Could you check a few things on this model? Use its own coordinates, in mm. A direction names the side the tool comes from. Give positions to 0.01 mm unless a question says otherwise; leave off trailing zeros. Loops run counter-clockwise (first coordinate to the right, second up) from the corner with the lowest first, then second, coordinate; pieces in that order, holes last. Notation, with made-up numbers: (19.25, 52) - (55.25, 52) arc R31 cw to (55.25, 86) - close; hole circle Ø5 at (47, 1.25). An arc over 180 degrees is marked (long way). Use CSV: the item, a comma, the result in double quotes.
from build123d import *

# Parameters (mm, degrees)
SZKIC1_W                                = 77
SZKIC1_H                                = 40
SZKIC1_R                                = 1.5
DODANIE_WYCI_GNI_CIE1_DEPTH             = 2
SZKIC2_W                                = 77
SZKIC2_H                                = 40
SZKIC2_W_2                              = 73
SZKIC2_H_2                              = 36
DODANIE_WYCI_GNI_CIE2_DEPTH             = 19
WYTNIJ_WYCI_GNI_CIE1_DEPTH              = 60.356970947
ZAOKR_GLENIE1_R                         = 2.5
SZKIC4_W                                = 77
SZKIC4_H                                = 1
DODANIE_WYCI_GNI_CIE3_DEPTH             = 10
SZKIC5_W                                = 6
SZKIC5_H                                = 10
DODANIE_WYCI_GNI_CIE4_DEPTH             = 5
ZAOKR_GLENIE2_R                         = 2.5
ZAOKR_GLENIE2_OF_LUSTRO1_R              = 2.5
LUSTRO2_START                           = -13
LUSTRO2_DEPTH                           = 6
LUSTRO2_START_2                         = 7
LUSTRO2_2_DEPTH                         = 6
DODANIE_WYCI_GNI_CIE5_REACH             = 50.2
SZKIC6_R                                = 8.7
DODANIE_WYCI_GNI_CIE5_DIRECTION_2_REACH = 50.2
ZAOKR_GLENIE3_R                         = 0.5


# Read off the part's stored shape, not the designer's step: Lustro2
with BuildPart() as part:
    # Szkic1 → Dodanie-wyciągnięcie1 (new body)
    with BuildSketch(Plane(origin=(0, 0, 0), x_dir=(1, 0, 0), z_dir=(0, 1, 0))):
        Rectangle(SZKIC1_W, SZKIC1_H)
        with Locations(Location((27.5, 9.5, 0), (0, 0, 270))):
            Circle(SZKIC1_R, mode=Mode.SUBTRACT)
        with Locations(Location((27.5, -9.5, 0), (0, 0, 90))):
            Circle(SZKIC1_R, mode=Mode.SUBTRACT)
        with Locations(Location((-27.5, -9.5, 0), (0, 0, 270))):
            Circle(SZKIC1_R, mode=Mode.SUBTRACT)
        with Locations(Location((-27.5, 9.5, 0), (0, 0, 90))):
            Circle(SZKIC1_R, mode=Mode.SUBTRACT)
    extrude(amount=DODANIE_WYCI_GNI_CIE1_DEPTH)

    # Szkic2 → Dodanie-wyciągnięcie2 (add)
    with BuildSketch(Plane(origin=(0, 2, 0), x_dir=(1, 0, 0), z_dir=(0, 1, 0))):
        Rectangle(SZKIC2_W, SZKIC2_H)
        Rectangle(SZKIC2_W_2, SZKIC2_H_2, mode=Mode.SUBTRACT)
    extrude(amount=DODANIE_WYCI_GNI_CIE2_DEPTH)

    # Szkic3 → Wytnij-wyciągnięcie1 (cut, through all)
    with BuildSketch(Plane.XY.offset(20)):
        Polygon((-12.5, 7.396479256), (12.5, 7.396479256), (12.5, 12.396479256), (25.5, 12.396479256), (25.5, 17.396479256), (36.5, 17.396479256), (36.5, 21), (-36.5, 21), (-36.5, 17.396479256), (-25.5, 17.396479256), (-25.5, 12.396479256), (-12.5, 12.396479256), align=None)
    extrude(amount=-WYTNIJ_WYCI_GNI_CIE1_DEPTH, mode=Mode.SUBTRACT)

    # Zaokrąglenie1
    zaokr_glenie1_edges = [part.edges().sort_by_distance(p)[0] for p in [
        (36.5, 17.396479256, 19),
        (25.5, 17.396479256, 19),
        (25.5, 12.396479256, 19),
        (12.5, 12.396479256, 19),
        (12.5, 7.396479256, 19),
        (-36.5, 17.396479256, 19),
        (-25.5, 17.396479256, 19),
        (-25.5, 12.396479256, 19),
        (-12.5, 12.396479256, 19),
        (-12.5, 7.396479256, 19),
        (12.5, 7.396479256, -19),
        (12.5, 12.396479256, -19),
        (25.5, 12.396479256, -19),
        (36.5, 17.396479256, -19),
        (25.5, 17.396479256, -19),
        (-12.5, 7.396479256, -19),
        (-12.5, 12.396479256, -19),
        (-36.5, 17.396479256, -19),
        (-25.5, 17.396479256, -19),
        (-25.5, 12.396479256, -19),
    ]]
    fillet(zaokr_glenie1_edges, radius=ZAOKR_GLENIE1_R - 0.0001)  # a hair under: the kernel refuses the full size

    # Szkic4 → Dodanie-wyciągnięcie3 (add)
    with BuildSketch(Plane(origin=(0, 2, 0), x_dir=(1, 0, 0), z_dir=(0, 1, 0))):
        Rectangle(SZKIC4_W, SZKIC4_H)
    extrude(amount=DODANIE_WYCI_GNI_CIE3_DEPTH)

    # Szkic5 → Dodanie-wyciągnięcie4 (add)
    with BuildSketch(Plane(origin=(-36.5, 0, 0), x_dir=(0, 0, -1), z_dir=(1, 0, 0))):
        with Locations((-10, 9.5)):
            Rectangle(SZKIC5_W, SZKIC5_H)
    dodanie_wyci_gni_cie4 = extrude(amount=DODANIE_WYCI_GNI_CIE4_DEPTH)

    # Zaokrąglenie2
    zaokr_glenie2_edges = [part.edges().sort_by_distance(p)[0] for p in [
        (-31.5, 14.5, 10),
    ]]
    fillet(zaokr_glenie2_edges, radius=ZAOKR_GLENIE2_R)

    # Lustro1: Dodanie-wyciągnięcie4 across plane
    add(dodanie_wyci_gni_cie4.mirror(Plane.XY))

    # Zaokrąglenie2 of Lustro1
    zaokr_glenie2_of_lustro1_edges = [part.edges().sort_by_distance(p)[0] for p in [
        (-31.5, 14.5, -10),
    ]]
    fillet(zaokr_glenie2_of_lustro1_edges, radius=ZAOKR_GLENIE2_OF_LUSTRO1_R)

    # Lustro2 outline → Lustro2 (add)
    with BuildSketch(Plane.XY.offset(LUSTRO2_START)):
        with BuildLine():
            Line((36.5, 14.5), (34, 14.5))
            ThreePointArc((34, 14.5), (32.232233047, 13.767766953), (31.5, 12))
            Line((31.5, 12), (31.5, 4.5))
            Line((31.5, 4.5), (36.5, 4.5))
            Line((36.5, 4.5), (36.5, 14.5))
        make_face()
    extrude(amount=LUSTRO2_DEPTH)

    # Lustro2 2 outline → Lustro2 2 (add)
    with BuildSketch(Plane.XY.offset(LUSTRO2_START_2)):
        with BuildLine():
            Line((36.5, 14.5), (34, 14.5))
            ThreePointArc((34, 14.5), (32.232233047, 13.767766953), (31.5, 12))
            Line((31.5, 12), (31.5, 4.5))
            Line((31.5, 4.5), (36.5, 4.5))
            Line((36.5, 4.5), (36.5, 14.5))
        make_face()
    extrude(amount=LUSTRO2_2_DEPTH)

    # Dodanie-wyciągnięcie5: up to this face of the body (flat: up to its plane)
    dodanie_wyci_gni_cie5_end = Plane(part.part.faces().sort_by_distance((31.5, 8.25, 10))[0])
    # Szkic6 → Dodanie-wyciągnięcie5 (add, up to the picked face)
    with BuildSketch(Plane(origin=(0, 0, 0), x_dir=(0, 0, -1), z_dir=(1, 0, 0)), mode=Mode.PRIVATE) as dodanie_wyci_gni_cie5_sk1:
        with Locations(Location((-9.25, 11, 0), (0, 0, 180))):
            Circle(SZKIC6_R)
    dodanie_wyci_gni_cie5_tool1 = split(extrude(dodanie_wyci_gni_cie5_sk1.sketch, amount=DODANIE_WYCI_GNI_CIE5_REACH, mode=Mode.PRIVATE), bisect_by=dodanie_wyci_gni_cie5_end, keep=Keep.BOTH, mode=Mode.PRIVATE)
    # Szkic6 → Dodanie-wyciągnięcie5 (add, up to the picked face)
    with BuildSketch(Plane(origin=(0, 0, 0), x_dir=(0, 0, -1), z_dir=(1, 0, 0)), mode=Mode.PRIVATE) as dodanie_wyci_gni_cie5_sk2:
        with Locations(Location((9.25, 11, 0), (0, 0, 180))):
            Circle(SZKIC6_R)
    dodanie_wyci_gni_cie5_tool2 = split(extrude(dodanie_wyci_gni_cie5_sk2.sketch, amount=DODANIE_WYCI_GNI_CIE5_REACH, mode=Mode.PRIVATE), bisect_by=dodanie_wyci_gni_cie5_end, keep=Keep.BOTH, mode=Mode.PRIVATE)
    add(dodanie_wyci_gni_cie5_tool1.solids().sort_by(Axis((0, 11, 9.25), (1, 0, 0)))[0])
    add(dodanie_wyci_gni_cie5_tool2.solids().sort_by(Axis((0, 11, -9.25), (1, 0, 0)))[0])

    # Dodanie-wyciągnięcie5 direction 2: up to this face of the body (flat: up to its plane)
    dodanie_wyci_gni_cie5_direction_2_end = Plane(part.part.faces().sort_by_distance((-31.5, 8.25, 10))[0])
    # Szkic6 → Dodanie-wyciągnięcie5 direction 2 (add, up to the picked face)
    with BuildSketch(Plane(origin=(0, 0, 0), x_dir=(0, 0, -1), z_dir=(1, 0, 0)), mode=Mode.PRIVATE) as dodanie_wyci_gni_cie5_direction_2_sk1:
        with Locations(Location((-9.25, 11, 0), (0, 0, 180))):
            Circle(SZKIC6_R)
    dodanie_wyci_gni_cie5_direction_2_tool1 = split(extrude(dodanie_wyci_gni_cie5_direction_2_sk1.sketch, amount=-DODANIE_WYCI_GNI_CIE5_DIRECTION_2_REACH, mode=Mode.PRIVATE), bisect_by=dodanie_wyci_gni_cie5_direction_2_end, keep=Keep.BOTH, mode=Mode.PRIVATE)
    # Szkic6 → Dodanie-wyciągnięcie5 direction 2 (add, up to the picked face)
    with BuildSketch(Plane(origin=(0, 0, 0), x_dir=(0, 0, -1), z_dir=(1, 0, 0)), mode=Mode.PRIVATE) as dodanie_wyci_gni_cie5_direction_2_sk2:
        with Locations(Location((9.25, 11, 0), (0, 0, 180))):
            Circle(SZKIC6_R)
    dodanie_wyci_gni_cie5_direction_2_tool2 = split(extrude(dodanie_wyci_gni_cie5_direction_2_sk2.sketch, amount=-DODANIE_WYCI_GNI_CIE5_DIRECTION_2_REACH, mode=Mode.PRIVATE), bisect_by=dodanie_wyci_gni_cie5_direction_2_end, keep=Keep.BOTH, mode=Mode.PRIVATE)
    add(dodanie_wyci_gni_cie5_direction_2_tool1.solids().sort_by(Axis((0, 11, 9.25), (-1, 0, 0)))[0])
    add(dodanie_wyci_gni_cie5_direction_2_tool2.solids().sort_by(Axis((0, 11, -9.25), (-1, 0, 0)))[0])

    # Zaokrąglenie3
    zaokr_glenie3_edges = [part.edges().sort_by_distance(p)[0] for p in [
        (-31.5, 11, 0.55),
        (31.5, 11, 0.55),
        (31.5, 11, -17.95),
        (-31.5, 11, -17.95),
    ]]
    fillet(zaokr_glenie3_edges, radius=ZAOKR_GLENIE3_R)


solid = part.part
1) Which directions (+Z, -Z, +X, -X, +Y, -Y) give clear straight access to the entire face, cutting with the end or side of a thin tool? Please do faces 1 (the flat face through (35, 14.5, -10)), 2 (the cylindrical face through (-35.79, 18.15, -19.01)), 3 (the flat face through (37, 21, 0)), 4 (the cylindrical face through (26.21, 16.64, 18.99)), 5 (the cylindrical face through (-13.25, 11.68, -19.01)).
Answer below:
face 1,"+Y"
face 2,"+Z, -Z, +Y"
face 3,"+Z, -Z, +X, -X, +Y"
face 4,"+Z, +Y"
face 5,"-Z, +Y"
2) Suppose I cut it at D-D (y = 16). State how many separate pieces and enclosed holes the cut face has, plus the area to 3 significant figures.
Answer below:
separate pieces,"4"
enclosed holes,"0"
area,"2,040 mm2"
3) Suppose I cut it at A-A (x = 7.5). Please give me the cut outline in (y, z), plus the area to 3 significant figures.
Answer below:
outline,"(0, -20) - (7.4, -20) - (7.4, -18) - (2, -18) - (2, -0.5) - (12, -0.5) - (12, 0.5) - (2, 0.5) - (2, 18) - (7.4, 18) - (7.4, 20) - (0, 20) - close; circle Ø17.4 at (11, -9.25); circle Ø17.4 at (11, 9.25)"
area,"587 mm2"
4) Suppose I cut it at C-C (x = 17.5). Please give me the cut outline in (y, z).
Answer below:
outline,"(0, -20) - (12.4, -20) - (12.4, -18) - (2, -18) - (2, -0.5) - (12, -0.5) - (12, 0.5) - (2, 0.5) - (2, 18) - (12.4, 18) - (12.4, 20) - (0, 20) - close; circle Ø17.4 at (11, -9.25); circle Ø17.4 at (11, 9.25)"
5) I'm going to push flat-ended pins straight in: P1, Ø1, axis at x = -31, z = 18.5, coming from the +Y side; P2, Ø2, axis at x = 18, z = 19, coming from the +Y side; P3, Ø1, axis at x = -2.5, z = -19.5, coming from the +Y side. Where does each tip first touch, or does it pass through?
Answer below:
P1,"stops at y = 17.4"
P2,"stops at y = 12.4"
P3,"stops at y = 7.4"
6) I need wall thicknesses on line 1 along X through (y, z) = (16.75, 14.5); line 2 along X through (y, z) = (1.25, -9.5); line 3 along Z through (x, y) = (-4.5, 5.75). Which ranges of each line are inside material? Lowest first, please.
Answer below:
line 1,"x = -38.5 to -36.5, -31.5 to 31.5, 36.5 to 38.5"
line 2,"x = -38.5 to -29, -26 to 26, 29 to 38.5"
line 3,"z = -20 to -18, -16.19 to -2.31, -0.5 to 0.5, 2.31 to 16.19, 18 to 20"
